from build123d import *

# Parameters (mm, degrees)
F0_W      = 234.762548
F0_H      = 46.762416
F0_W_2    = 230.000048
F0_H_2    = 41.999916
F1_DEPTH  = 6.35
F2_W      = 234.762548
F2_H      = 46.762416
F2_W_2    = 217.300048
F2_H_2    = 29.299916
F3_DEPTH  = 2.38125
F4_R      = 3.96875
F5_DEPTH  = 8.73125
F6_R      = 7.9375
F7_R      = 2.15265
F8_DEPTH  = 8.73125
F9_R      = 0.79375
F10_DEPTH = 6.35


with BuildPart() as f1:
    # F0 (on Top) → F1 (new body)
    with BuildSketch(Plane.XY):
        Rectangle(F0_W, F0_H)
        Rectangle(F0_W_2, F0_H_2, mode=Mode.SUBTRACT)
    extrude(amount=F1_DEPTH)

    # F2 (on face) → F3 (join)
    with BuildSketch(Plane(origin=(0, 0, 0), x_dir=(1, 0, 0), z_dir=(0, 0, -1))):
        Rectangle(F2_W, F2_H)
        Rectangle(F2_W_2, F2_H_2, mode=Mode.SUBTRACT)
    extrude(amount=F3_DEPTH)

    # F4 (on face) → F5 (join, through all)
    with BuildSketch(Plane.XY.offset(6.35)):
        with Locations((118.36762, 24.367554)):
            Circle(F4_R)
        with Locations((118.36762, -24.367554)):
            Circle(F4_R)
        with Locations((-118.36762, -24.367554)):
            Circle(F4_R)
        with Locations((-118.36762, 24.367554)):
            Circle(F4_R)
    extrude(amount=-F5_DEPTH)

    # F6
    f6_edges = [f1.edges().sort_by_distance(p)[0] for p in [
        (114.523391, 23.381208, 1.984375),
        (117.381274, 20.523325, 1.984375),
        (117.381274, -20.523325, 1.984375),
        (114.523391, -23.381208, 1.984375),
        (-117.381274, -20.523325, 1.984375),
        (-114.523391, -23.381208, 1.984375),
        (-114.523391, 23.381208, 1.984375),
        (-117.381274, 20.523325, 1.984375),
    ]]
    fillet(f6_edges, radius=F6_R)

    # F7 (on face) → F8 (cut, through all)
    with BuildSketch(Plane.XY.offset(6.35)):
        with Locations((118.36762, 24.367554)):
            Circle(F7_R)
        with Locations((118.36762, -24.367554)):
            Circle(F7_R)
        with Locations((-118.36762, 24.367554)):
            Circle(F7_R)
        with Locations((-118.36762, -24.367554)):
            Circle(F7_R)
    extrude(amount=-F8_DEPTH, mode=Mode.SUBTRACT)

    # F9 (on face) → F10 (cut, through all)
    with BuildSketch(Plane.XY.offset(6.35)):
        with Locations((-115.000024, 20.999958)):
            Circle(F9_R)
        with Locations((-115.000024, -20.999958)):
            Circle(F9_R)
        with Locations((115.000024, 20.999958)):
            Circle(F9_R)
        with Locations((115.000024, -20.999958)):
            Circle(F9_R)
    extrude(amount=-F10_DEPTH, mode=Mode.SUBTRACT)


solid = f1.part
Geometry check sheet. Reference: the model listing, model coordinates, mm. A direction names the side the tool comes from. Give positions to 0.01 mm unless a question says otherwise; leave off trailing zeros. Order: outer loops, then holes, each group sorted by start corner. A loop starts at its lowest first (then second) coordinate and runs counter-clockwise, first axis right, second up. Notation, with made-up numbers: (-18, 62) - (-9, 62) arc R27 cw to (-9, 94) - close; hole circle Ø2 at (76.5, -34). An arc over 180 degrees is marked (long way). Use one line per item in the form item = value.
1) Access from +Z, -Z, +X, -X, +Y, -Y to the whole of each face (thin tool, end or side, straight path). Record for faces 1 (the face through (-112.275, 24.231, 2.045)), 2 (the face through (-115, 0, 3)), 3 (the face through (-118.28, 18.37, 2.05)), 4 (the face through (-112.37, -24.28, 2.05)), 5 (the face through (-120.52, 24.46, 2.05)).
Working result:
face_1 = +Z, -Z, +Y
face_2 = +Z
face_3 = +Z, -Z, -X
face_4 = +Z, -Z, -Y
face_5 = +Z, -Z
2) Sectioned sample at B-B (y = -8). Record the boundary of the cut face in (x, z), and give its area (3 significant figures).
Working result:
outline = (-117.38, -2.38) - (-108.65, -2.38) - (-108.65, 0) - (-115, 0) - (-115, 6.35) - (-117.38, 6.35) - close; (108.65, -2.38) - (117.38, -2.38) - (117.38, 6.35) - (115, 6.35) - (115, 0) - (108.65, 0) - close
area = 71.8 mm^2
3) Sectioned sample at A-A (x = -15). Record the boundary of the cut face in (y, z).
Working result:
outline = (-23.38, -2.38) - (-14.65, -2.38) - (-14.65, 0) - (-21, 0) - (-21, 6.35) - (-23.38, 6.35) - close; (14.65, -2.38) - (23.38, -2.38) - (23.38, 6.35) - (21, 6.35) - (21, 0) - (14.65, 0) - close
4) Material ranges on probe 1 along Y at (x, z) = (-99, 3.75); probe 2 along X at (y, z) = (-11, 4); probe 3 along X at (y, z) = (-25, 5.25), recorded low to high. Write a range as from..to.
Working result:
probe_1 = -23.38..-21, 21..23.38
probe_2 = -117.38..-115, 115..117.38
probe_3 = -122.29..-120.43, -116.31..-113.51, 113.51..116.31, 120.43..122.29
5) Sectioned sample at C-C (z = 2.5). Record the boundary of the cut face in (x, y) (1 decimal), and give its area (3 significant figures).
Working result:
outline = (-120.7, -21.1) arc R4 ccw (long way) to (-115.1, -26.7) arc R7.9 cw to (-108.7, -23.4) - (108.7, -23.4) arc R7.9 cw to (115.1, -26.7) arc R4 ccw (long way) to (120.7, -21.1) arc R7.9 cw to (117.4, -14.7) - (117.4, 14.7) arc R7.9 cw to (120.7, 21.1) arc R4 ccw (long way) to (115.1, 26.7) arc R7.9 cw to (108.7, 23.4) - (-108.7, 23.4) arc R7.9 cw to (-115.1, 26.7) arc R4 ccw (long way) to (-120.7, 21.1) arc R7.9 cw to (-117.4, 14.7) - (-117.4, -14.7) arc R7.9 cw to start; hole circle Ø4.3 at (-118.4, -24.4); hole circle Ø4.3 at (-118.4, 24.4); hole (-115, -20.2) arc R0.8 ccw (long way) to (-114.2, -21) - (114.2, -21) arc R0.8 ccw (long way) to (115, -20.2) - (115, 20.2) arc R0.8 ccw (long way) to (114.2, 21) - (-114.2, 21) arc R0.8 ccw (long way) to (-115, 20.2) - close; hole circle Ø4.3 at (118.4, -24.4); hole circle Ø4.3 at (118.4, 24.4)
area = 1,470 mm^2
6) Depth check by flat-ended pin: pin 1 Ø2.5 at (y, z) = (5, -1.5) entering from -X; pin 2 Ø1.4 at (x, y) = (115, -21) entering from +Z; pin 3 Ø1.2 at (y, z) = (0.5, -1) entering from +X; pin 4 Ø7 at (x, y) = (118.37, -24.37) entering from +Z. Enter the tip coordinate at first touch or a pass-through.
Working result:
pin_1 = -117.38
pin_2 = 0
pin_3 = 117.38
pin_4 = 6.35
7) Draft check along X on faces 6 (the face through (-118.231, -18.275, 2.045)), 7 (the face through (112.275, -24.231, 2.045)), 8 (the face through (18, 23, 6.35)). Enter one of: released by +X, released by -X, zero draft, split by the parting line, or undercut.
Working result:
face_6 = released by -X
face_7 = undercut
face_8 = zero draft
